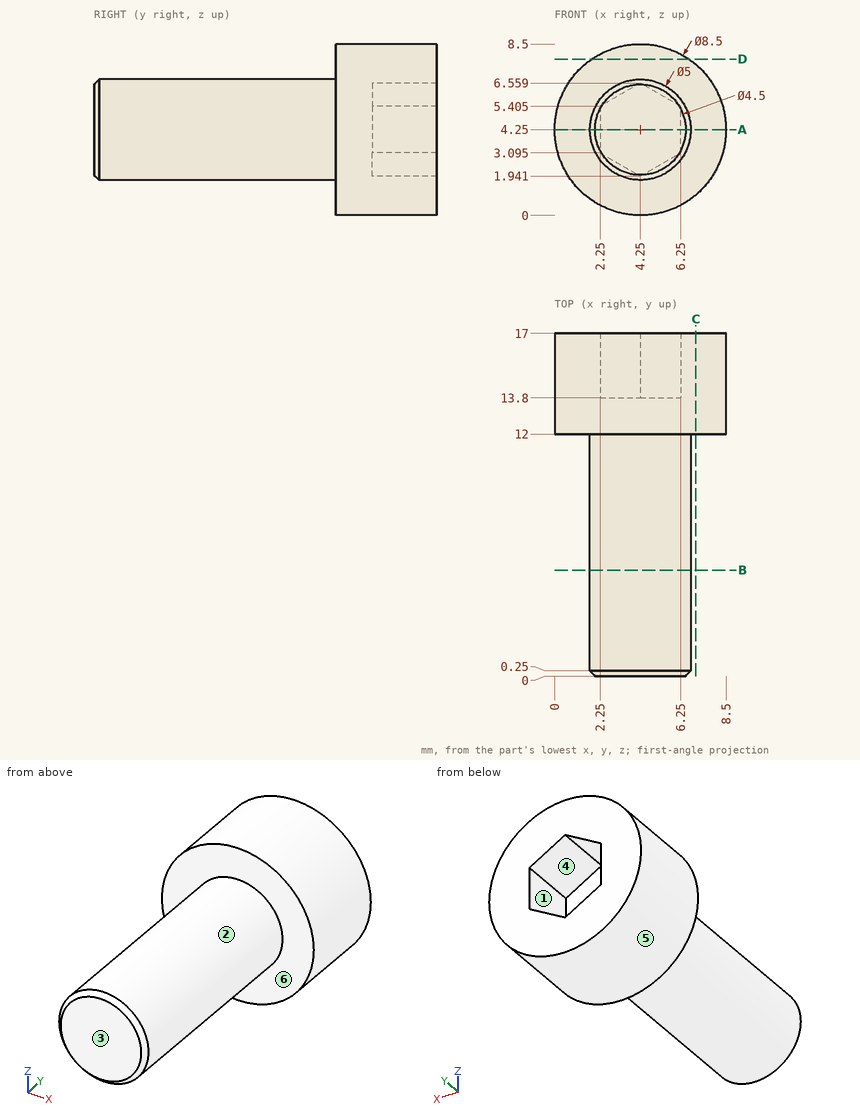
Here's the drawing with two shaded views (mm, measured from the low corner). I have some questions. A direction names the side the tool comes from. Round coordinates to 2 decimals unless told otherwise and drop trailing zeros. Order: outer loops, then holes, each group sorted by start corner. A loop starts at its lowest first (then second) coordinate and runs counter-clockwise, first axis right, second up. Notation, with made-up numbers: M 71,65 L 126,65 A18 ccw 126,75 Z; hole C 81.5,47.5 d1. An arc over 180 degrees is marked long. Use CSV: the item, a comma, the result in double quotes.
1) On a 3-axis mill with a long thin cutter (end or side, diameter ignored), from which of +Z, -Z, +X, -X, +Y, -Y can I reach the whole of each face in a straight line? I mean the marked faces 5 and 6. Say none if no direction works.
Taken from the geometry:
face 5,"+Y, -Y"
face 6,"-Y"
2) I want a section at A-A (z = 4.25). List the corners of the cut face in (x, y) for me.
Taken from the geometry:
outline,"M 0,12 L 1.75,12 L 1.75,0.25 L 2,0 L 6.5,0 L 6.75,0.25 L 6.75,12 L 8.5,12 L 8.5,17 L 6.25,17 L 6.25,13.8 L 2.25,13.8 L 2.25,17 L 0,17 Z"
3) I want a section at C-C (x = 7). List the corners of the cut face in (y, z) for me.
Taken from the geometry:
outline,"M 12,1.01 L 17,1.01 L 17,7.49 L 12,7.49 Z"
4) I need wall thicknesses on line 1 along Y through (x, z) = (6, 4.25); line 2 along X through (y, z) = (14.75, 5); line 3 along Y through (x, z) = (1.25, 4). Which ranges of each line are inside material? Lowest first, please. Write a range as [from, to].
Taken from the geometry:
line 1,"[0, 13.8]"
line 2,"[0.07, 2.25], [6.25, 8.43]"
line 3,"[12, 17]"
5) If we mould it in two halves opening along Z, with no side actions, what happens to the marked faces 1, 2, 3 and 4? For each: pulls with the +Z half, pulls with the -Z half, needs draft (parallel to the pull), parting line crosses it, or undercut.
Taken from the geometry:
face 1,"undercut"
face 2,"parting line crosses it"
face 3,"needs draft"
face 4,"undercut"
6) I want a section at D-D (z = 7.75). List the corners of the cut face in (x, y) for me, then the cut area to 3 significant figures.
Taken from the geometry:
outline,"M 1.84,12 L 6.66,12 L 6.66,17 L 1.84,17 Z"
area,"24.1 mm^2"
7) I want a section at B-B (y = 5.25). List the corners of the cut face in (x, z) for me, then the cut area to 3 significant figures.
Taken from the geometry:
outline,"C 4.25,4.25 d5"
area,"19.6 mm^2"
8) I'm going to push flat-ended pins straight in: P1, Ø3, axis at x = 1, y = 6, coming from the -Z side (1 decimal); P2, Ø5, axis at y = 5.5, z = 7, coming from the -X side; P3, Ø4, axis at x = 7.5, y = 15, coming from the -Z side; P4, Ø1, axis at x = 2.5, z = 6, coming from the -Y side. Where does each tip first touch, or does it pass through?
Taken from the geometry:
P1,"z = 2.5"
P2,"x = 1.76"
P3,"z = 0.19"
P4,"y = 0"
